from build123d import *

# Parameters (mm, degrees)
SKETCH2_R           = 6.35
BOSS_EXTRUDE1_DEPTH = 30
SKETCH3_R           = 20
BOSS_EXTRUDE3_DEPTH = 10
FILLET1_R           = 3.9
SKETCH4_R           = 20
SKETCH4_R_2         = 16.85
BOSS_EXTRUDE4_DEPTH = 25
FILLET2_R           = 2.5
FILLET3_R           = 2.5
SKETCH5_R           = 2.5796875
CUT_EXTRUDE1_DEPTH  = 71.887234394


with BuildPart() as part:
    # Sketch1 → Revolve3 (revolve)
    with BuildSketch(Plane(origin=(0, 0, 0), x_dir=(1, 0, 0), z_dir=(0, 1, 0))):
        with BuildLine():
            Line((0, 16.75), (0, -16.75))
            ThreePointArc((0, -16.75), (16.75, 0), (0, 16.75))
        make_face()
    revolve(axis=Axis((0, 0, -16.75), (0, 0, 1)))

    # Sketch2 → Boss-Extrude1 (add)
    with BuildSketch(Plane(origin=(0, 0, 0), x_dir=(1, 0, 0), z_dir=(0, 1, 0))):
        with Locations(Location((0, 0, 0), (0, 0, 90))):
            Circle(SKETCH2_R)
    extrude(amount=BOSS_EXTRUDE1_DEPTH)

    # Sketch3 → Boss-Extrude3 (add)
    with BuildSketch(Plane(origin=(0, 30, 0), x_dir=(1, 0, 0), z_dir=(0, 1, 0))):
        with Locations(Location((0, 0, 0), (0, 0, 270))):
            Circle(SKETCH3_R)
    extrude(amount=BOSS_EXTRUDE3_DEPTH)

    # Fillet1
    fillet1_edges = [part.edges().sort_by_distance(p)[0] for p in [
        (0, 30, 6.35),
    ]]
    fillet(fillet1_edges, radius=FILLET1_R)

    # Sketch4 → Boss-Extrude4 (add)
    with BuildSketch(Plane(origin=(0, 40, 0), x_dir=(1, 0, 0), z_dir=(0, 1, 0))):
        with Locations(Location((0, 0, 0), (0, 0, 270))):
            Circle(SKETCH4_R)
        with Locations(Location((0, 0, 0), (0, 0, 270))):
            Circle(SKETCH4_R_2, mode=Mode.SUBTRACT)
    extrude(amount=BOSS_EXTRUDE4_DEPTH)

    # Fillet2
    fillet2_edges = [part.edges().sort_by_distance(p)[0] for p in [
        (0, 30, -20),
    ]]
    fillet(fillet2_edges, radius=FILLET2_R)

    # Fillet3
    fillet3_edges = [part.edges().sort_by_distance(p)[0] for p in [
        (0, 15.499677416, 6.35),
    ]]
    fillet(fillet3_edges, radius=FILLET3_R)

    # Sketch5 → Cut-Extrude1 (cut, through all)
    with BuildSketch(Plane.XY):
        with Locations(Location((0, 52.7, 0), (0, 0, 90.000000055))):
            Circle(SKETCH5_R)
    extrude(amount=CUT_EXTRUDE1_DEPTH, mode=Mode.SUBTRACT)


solid = part.part
CAD build for the part. Positions are in the model's coordinates, mm. A direction names the side the tool comes from. Round coordinates to 2 decimals unless told otherwise and drop trailing zeros. Write each loop counter-clockwise with the first axis right and the second up, starting at its lowest first coordinate (ties: lowest second). Pieces come first, ordered by that corner, then holes.
(1) Slice it at A-A, the plane y = 52.7. Write the cut outline in (x, z).
(2) Probe line 1 along X through (y, z) = (59, 0); line 2 along Y through (x, z) = (0, 17); line 3 along Z through (x, y) = (-4, 43.5). List the from-to ranges inside material, lowest first.
(3) Mould opens along Y. For faces 1 (the face through (-8, 30, 8)), 2 (the face through (3.86, 21.53, 5.04)), 3 (the face through (-15, 65, -9)) say: pulls with the +Y half, pulls with the -Y half, needs draft (parallel to the pull), parting line crosses it, or undercut.
(4) Drop flat-ended pins along their axis: P1, Ø2, axis at x = 5, y = -8, coming from the -Z side; P2, Ø10, axis at y = 39.5, z = -8, coming from the +X side; P3, Ø2, axis at x = -6.5, z = -9.5, coming from the +Y side. Give the stop position or say it passes through.
(5) Slice it at B-B, the plane y = 10.5. Write the cut outline in (x, z), and give its area (3 significant figures).
(6) 3-axis set-ups, long thin cutter, end or side, ignore diameter. For faces 4 (the face through (-19.524, 48.522, -4.336)), 5 (the face through (-0.113, 50.123, 18.302)), 6 (the face through (16.707, 52.325, -2.194)): which of +Z, -Z, +X, -X, +Y, -Y reach the whole face in a straight line?
From the geometry:
1. outline: (-2.58, 16.65) - (-2.58, 19.83) arc R20 ccw (long way) to (2.58, 19.83) - (2.58, 16.65) arc R16.85 cw (long way) to start
2. line 1: x = -20 to -16.85, 16.85 to 20
2. line 2: y = 30 to 50.12, 55.28 to 65
2. line 3: z = -19.6 to -16.37, 16.37 to 19.6
3. face 1: undercut
3. face 2: undercut
3. face 3: pulls with the +Y half
4. P1: stops at z = -14.47
4. P2: stops at x = 19.77
4. P3: stops at y = 40
5. outline: circle Ø26.1 at (0, 0)
5. area: 535 mm2
6. face 4: +Y, -Y
6. face 5: +Z
6. face 6: +Y
